from build123d import *
from OCP.BRepFilletAPI import BRepFilletAPI_MakeChamfer

# Parameters (mm, degrees)
SKETCH_1_R           = 1.5
SKETCH_1_W           = 16.5
SKETCH_1_H           = 10
EXTRUDE_1_DEPTH      = 3
SKETCH_2_W           = 55
SKETCH_2_H           = 46
SKETCH_2_W_2         = 49
SKETCH_2_H_2         = 40
EXTRUDE_2_DEPTH      = 30
SKETCH_3_W           = 22.4
SKETCH_3_H           = 13.1
CUT_EXTRUDE_1_DEPTH  = 40
EXTRUDE_3_DEPTH      = 12.9
EXTRUDE_3_DEPTH_BACK = 2
FILLET_1_R           = 4
CHAMFER_1_SIZE       = 1.5
CHAMFER_1_SIZE2      = 5
CHAMFER_2_SIZE       = 5
CHAMFER_2_SIZE2      = 1.5
CHAMFER_3_SIZE       = 5
CHAMFER_3_SIZE_2     = 3
CHAMFER_6_SIZE       = 6
CHAMFER_6_SIZE2      = 5
FILLET_2_R           = 3
FILLET_3_R           = 2


# Some blends are built 0.0001 mm under size
with BuildPart() as part:
    # Эскиз1 → Бобышка-Вытянуть1 (new body)
    with BuildSketch(Plane.XY):
        Polygon((27.5, 43), (-27.5, 43), (-27.5, -3), (-27.5, -18), (-21.5, -18), (-21.5, -3), (21.5, -3), (21.5, -18), (27.5, -18), (27.5, -3), align=None)
        with Locations((-24.5, -13)):
            Circle(SKETCH_1_R, mode=Mode.SUBTRACT)
        with Locations((24.5, -13)):
            Circle(SKETCH_1_R, mode=Mode.SUBTRACT)
        with Locations((0, 35)):
            Rectangle(SKETCH_1_W, SKETCH_1_H, mode=Mode.SUBTRACT)
    extrude(amount=EXTRUDE_1_DEPTH)

    # Эскиз2 → Бобышка-Вытянуть2 (add)
    with BuildSketch(Plane.XY.offset(3)):
        with Locations((0, 20)):
            Rectangle(SKETCH_2_W, SKETCH_2_H)
        with Locations((0, 20)):
            Rectangle(SKETCH_2_W_2, SKETCH_2_H_2, mode=Mode.SUBTRACT)
    extrude(amount=EXTRUDE_2_DEPTH)

    # Эскиз3 → Вырез-Вытянуть1 (cut)
    with BuildSketch(Plane(origin=(0, 43, 0), x_dir=(1, 0, 0), z_dir=(0, 1, 0))):
        with Locations((0, -26.65)):
            Rectangle(SKETCH_3_W, SKETCH_3_H)
    extrude(amount=-CUT_EXTRUDE_1_DEPTH, mode=Mode.SUBTRACT)

    # Эскиз4 → Бобышка-Вытянуть3 (add, two sides: drawn at the far end of the back side and taken through both)
    with BuildSketch(Plane.XY.offset(20.1).offset(-EXTRUDE_3_DEPTH_BACK)):
        Polygon((11.2, 40), (11.2, 40.8), (11, 40.8), (9.45, 40.8), (9.45, 40), align=None)
        Polygon((11.2, 40), (9.45, 40), (9.45, 39.7), (11, 39.7), (11, 38), (9.45, 38), (9.45, 37), (12.95, 37), (12.95, 40), align=None)
        Polygon((-11.2, 40), (-9.45, 40), (-9.45, 40.8), (-11, 40.8), (-11.2, 40.8), align=None)
        Polygon((-9.45, 39.7), (-9.45, 40), (-11.2, 40), (-12.95, 40), (-12.95, 37), (-9.45, 37), (-9.45, 38), (-11, 38), (-11, 39.7), align=None)
    extrude(amount=EXTRUDE_3_DEPTH + EXTRUDE_3_DEPTH_BACK)

    # Скругление1
    # the kernel refuses this fillet: 4 mm, written as the material it adds along each edge
    with BuildSketch(Plane(origin=(-12.95, 40, 18.1), x_dir=(-1, 0, 0), z_dir=(0, 0, 1))) as fillet_1_piece_1:
        with BuildLine():
            CenterArc((3.872983346, 4), FILLET_1_R, 194.477512186, 75.522487814)
            Line((0, 3), (-0.077459667, 2.98))
            ThreePointArc((-0.077459667, 2.98), (-0.08, 1.5), (-0.08, 0))
            Line((-0.08, 0), (0, -0.08))
            Line((0, -0.08), (3.872983346, -0.08))
            Line((3.872983346, -0.08), (3.872983346, 0))
        make_face()
    extrude(amount=14.9)
    with BuildSketch(Plane(origin=(12.95, 40, 33), x_dir=(0, -1, 0), z_dir=(0, 0, -1))) as fillet_1_piece_2:
        with BuildLine():
            CenterArc((4, -3.872983346), FILLET_1_R, 104.477512186, 75.522487814)
            Line((0, -3.872983346), (-0.08, -3.872983346))
            Line((-0.08, -3.872983346), (-0.08, 0))
            Line((-0.08, 0), (0, 0.08))
            ThreePointArc((0, 0.08), (1.5, 0.08), (2.98, 0.077459667))
            Line((2.98, 0.077459667), (3, 0))
        make_face()
    extrude(amount=14.9)

    # Фаска1
    chamfer_1_edges = [part.edges().sort_by_distance(p)[0] for p in [
        (9.45, 37.5, 33),
        (-9.45, 40.25, 33),
        (-9.45, 37.5, 33),
    ]]
    chamfer_1_side = [part.faces().sort_by_distance(p)[0] for p in [
        (13.93441787, 39.729121995, 33),
    ]]
    chamfer(chamfer_1_edges, length=CHAMFER_1_SIZE, length2=CHAMFER_1_SIZE2, reference=chamfer_1_side[0])

    # Фаска2
    chamfer_2_edges = [part.edges().sort_by_distance(p)[0] for p in [
        (9.45, 40.25, 33),
    ]]
    chamfer_2_side = [part.faces().sort_by_distance(p)[0] for p in [
        (9.45, 40.233772819, 26.247768763),
    ]]
    chamfer(chamfer_2_edges, length=CHAMFER_2_SIZE, length2=CHAMFER_2_SIZE2, reference=chamfer_2_side[0])

    # Фаска3
    chamfer_3_edges_1 = [part.edges().sort_by_distance(p)[0] for p in [
        (13.136491673, 40, 18.1),
    ]]
    chamfer_3_side_1 = [part.faces().sort_by_distance(p)[0] for p in [
        (13.136491673, 40, 18.04),
    ]]
    chamfer_3_edges_2 = [part.edges().sort_by_distance(p)[0] for p in [
        (-13.136491673, 40, 18.1),
    ]]
    chamfer_3_side_2 = [part.faces().sort_by_distance(p)[0] for p in [
        (-13.136491673, 40, 18.04),
    ]]
    chamfer_3 = BRepFilletAPI_MakeChamfer(part.part.solid().wrapped)
    for e in chamfer_3_edges_1:
        chamfer_3.Add(CHAMFER_3_SIZE - 0.0001, CHAMFER_3_SIZE_2 - 0.0001, e.wrapped, chamfer_3_side_1[0].wrapped)
    for e in chamfer_3_edges_2:
        chamfer_3.Add(CHAMFER_3_SIZE - 0.0001, CHAMFER_3_SIZE_2 - 0.0001, e.wrapped, chamfer_3_side_2[0].wrapped)
    add(Compound.cast(chamfer_3.Shape()), mode=Mode.REPLACE)  # a hair under: the kernel refuses the full size

    # Фаска5
    # the kernel refuses this chamfer: 3, 2 mm, written as the material it takes off along each edge
    with BuildSketch(Plane(origin=(9.45, 41.988024108, 9.786682308), x_dir=(0, 0.8574959522145404, 0.514490711223904), z_dir=(0, -0.514490711223904, 0.8574959522145406))) as chamfer_5_piece_1_section:
        with BuildLine():
            Line((3.099846035, 0.066564024), (-0.099846035, -2.066564024))
            Line((-0.099846035, -2.066564024), (-0.159846035, -2.066564024))
            ThreePointArc((-0.159846035, -2.066564024), (-0.06, -1.033282012), (-0.06, 0))
            Line((-0.06, 0), (0, 0.06))
            ThreePointArc((0, 0.06), (1.549923018, 0.06), (3.099846035, 0.126564024))
            Line((3.099846035, 0.126564024), (3.099846035, 0.066564024))
        make_face()
    chamfer_5_piece_1 = extrude(amount=17.446278464, mode=Mode.PRIVATE)
    chamfer_5_piece_1 = split(chamfer_5_piece_1, bisect_by=Plane(origin=(9.45, 40, 9.786682308), z_dir=(0, -1, 0)), keep=Keep.TOP, mode=Mode.PRIVATE)
    add(chamfer_5_piece_1, mode=Mode.SUBTRACT)
    with BuildSketch(Plane(origin=(-9.45, 41.988024108, 9.786682308), x_dir=(-1, 0, 0), z_dir=(0, -0.514490711223904, 0.8574959522145406))) as chamfer_5_piece_2_section:
        with BuildLine():
            Line((2.066564024, 0.099846035), (-0.066564024, -3.099846035))
            Line((-0.066564024, -3.099846035), (-0.126564024, -3.099846035))
            ThreePointArc((-0.126564024, -3.099846035), (-0.06, -1.549923018), (-0.06, 0))
            Line((-0.06, 0), (0, 0.06))
            ThreePointArc((0, 0.06), (1.033282012, 0.06), (2.066564024, 0.159846035))
            Line((2.066564024, 0.159846035), (2.066564024, 0.099846035))
        make_face()
    chamfer_5_piece_2 = extrude(amount=17.446278464, mode=Mode.PRIVATE)
    chamfer_5_piece_2 = split(chamfer_5_piece_2, bisect_by=Plane(origin=(-9.45, 40, 9.786682308), z_dir=(0, -1, 0)), keep=Keep.TOP, mode=Mode.PRIVATE)
    add(chamfer_5_piece_2, mode=Mode.SUBTRACT)

    # Фаска6: one chamfer whose edges measure the first distance from different faces: ONE call of the kernel's chamfer builder (chamfer() names one face for all edges)
    chamfer_6_edges_1 = [part.edges().sort_by_distance(p)[0] for p in [
        (24.5, -3, 3),
    ]]
    chamfer_6_side_1 = [part.faces().sort_by_distance(p)[0] for p in [
        (24.5, -10.286914786, 3),
    ]]
    chamfer_6_edges_2 = [part.edges().sort_by_distance(p)[0] for p in [
        (-24.5, -3, 3),
    ]]
    chamfer_6_side_2 = [part.faces().sort_by_distance(p)[0] for p in [
        (-24.5, -10.286914786, 3),
    ]]
    chamfer_6 = BRepFilletAPI_MakeChamfer(part.part.solid().wrapped)
    for e in chamfer_6_edges_1:
        chamfer_6.Add(CHAMFER_6_SIZE, CHAMFER_6_SIZE2, e.wrapped, chamfer_6_side_1[0].wrapped)  # the first distance lies on this face
    for e in chamfer_6_edges_2:
        chamfer_6.Add(CHAMFER_6_SIZE, CHAMFER_6_SIZE2, e.wrapped, chamfer_6_side_2[0].wrapped)  # the first distance lies on this face
    add(Compound.cast(chamfer_6.Shape()), mode=Mode.REPLACE)

    # Скругление2
    fillet_2_edges = [part.edges().sort_by_distance(p)[0] for p in [
        (27.5, -18, 1.5),
        (21.5, -18, 1.5),
        (-21.5, -18, 1.5),
        (-27.5, -18, 1.5),
    ]]
    fillet(fillet_2_edges, radius=FILLET_2_R - 0.0001)  # a hair under: the kernel refuses the full size

    # Скругление3
    fillet_3_edges = [part.edges().sort_by_distance(p)[0] for p in [
        (-16.375, 40, 3),
        (16.375, 40, 3),
        (-24.5, 20, 3),
        (0, 0, 3),
        (24.5, 20, 3),
        (-24.5, 0, 18),
        (24.5, 0, 18),
        (24.5, 40, 18),
        (-24.5, 40, 18),
    ]]
    fillet(fillet_3_edges, radius=FILLET_3_R)


solid = part.part
Here's how the part is built. I have some questions about the finished solid (model axes, mm). A direction names the side the tool comes from. Round coordinates to 2 decimals unless told otherwise and drop trailing zeros. Order: outer loops, then holes, each group sorted by start corner. A loop starts at its lowest first (then second) coordinate and runs counter-clockwise, first axis right, second up. Notation, with made-up numbers: M 12,78 L 55,78 A18 cw 55,84 Z; hole C -33.5,68 d6. An arc over 180 degrees is marked long. One line per question, with ' | ' between items.
1) Imagine slicing it at B-B, the plane x = -6.5. Write out the boundary of the cut face in (y, z), plus the area to 3 significant figures.
Checked values:
outline: M -3,0 L 30,0 L 30,3 L 2,3 A2 cw 0,5 L 0,33 L -3,33 Z; M 40,0 L 43,0 L 43,20.1 L 40,20.1 Z | area: 250 mm²
2) On a 3-axis mill with a long thin cutter (end or side, diameter ignored), from which of +Z, -Z, +X, -X, +Y, -Y can I reach the whole of each face in a straight line? I mean faces 1 (the flat face through (0, 0, 19)), 2 (the flat face through (-10.677, 37.808, 19.007)), 3 (the flat face through (-10.2, 40.2, 30.5)). Say none if no direction works.
Checked values:
face 1: +Z | face 2: none | face 3: +Z, +Y
3) I need wall thicknesses on line 1 (X direction, y = 35, z = 5); line 2 (Y direction, x = -17, z = 31); line 3 (Y direction, x = 24.5, z = 2.2). Which ranges of each line are inside material? Lowest first, please.
Checked values:
line 1: x = -27.5 to -24.5, 24.5 to 27.5 | line 2: y = -3 to 0, 40 to 43 | line 3: y = -18 to -14.5, -11.5 to 43
4) We'd pull the mould along X, two halves only. Please class faces 4 (the cylindrical face through (-26.6, -17.14, 1.52)), 5 (the flat face through (0, 20, 3)), 6 (the flat face through (27.5, 20, 16)): released by +X, released by -X, zero draft, split by the parting line, or undercut.
Checked values:
face 4: released by -X | face 5: undercut | face 6: released by +X
5) Imagine slicing it at C-C, the plane x = -18. Write out the boundary of the cut face in (y, z), plus the area to 3 significant figures.
Checked values:
outline: M -3,0 L 43,0 L 43,33 L 40,33 L 40,5 A2 cw 38,3 L 2,3 A2 cw 0,5 L 0,33 L -3,33 Z | area: 320 mm²
6) Imagine slicing it at A-A, the plane y = -13. Write out the boundary of the cut face in (x, z), plus the area to 3 significant figures.
Checked values:
outline: M -27.5,0 L -26,0 L -26,3 L -27.5,3 Z; M -23,0 L -21.5,0 L -21.5,3 L -23,3 Z; M 21.5,0 L 23,0 L 23,3 L 21.5,3 Z; M 26,0 L 27.5,0 L 27.5,3 L 26,3 Z | area: 18.0 mm²
7) I'm going to push flat-ended pins straight in: pin 1 Ø12 at (x, z) = (-14, 18) entering from -Y; pin 2 Ø1.2 at (x, z) = (-10.5, 21.5) entering from +Y; pin 3 Ø6.5 at (x, y) = (-24, -13) entering from +Z. Where does each tip first touch, or does it pass through?
Checked values:
pin 1: stops at y = -3 | pin 2: stops at y = 40.8 | pin 3: stops at z = 3
